For this review, use the dimensioned drawing (mm, ordinates from the lowest corner) and the shaded views. A direction names the side the tool comes from. Round coordinates to 2 decimals unless told otherwise and drop trailing zeros. Write each loop counter-clockwise with the first axis right and the second up, starting at its lowest first coordinate (ties: lowest second). Pieces come first, ordered by that corner, then holes. Notation, with made-up numbers: M 63.25,37 L 75.25,37 A27 cw 75.25,54 Z; hole C 51,-32.5 d6. An arc over 180 degrees is marked long. Write each question's results on one line, items separated by ' | '. Start each with the question number.
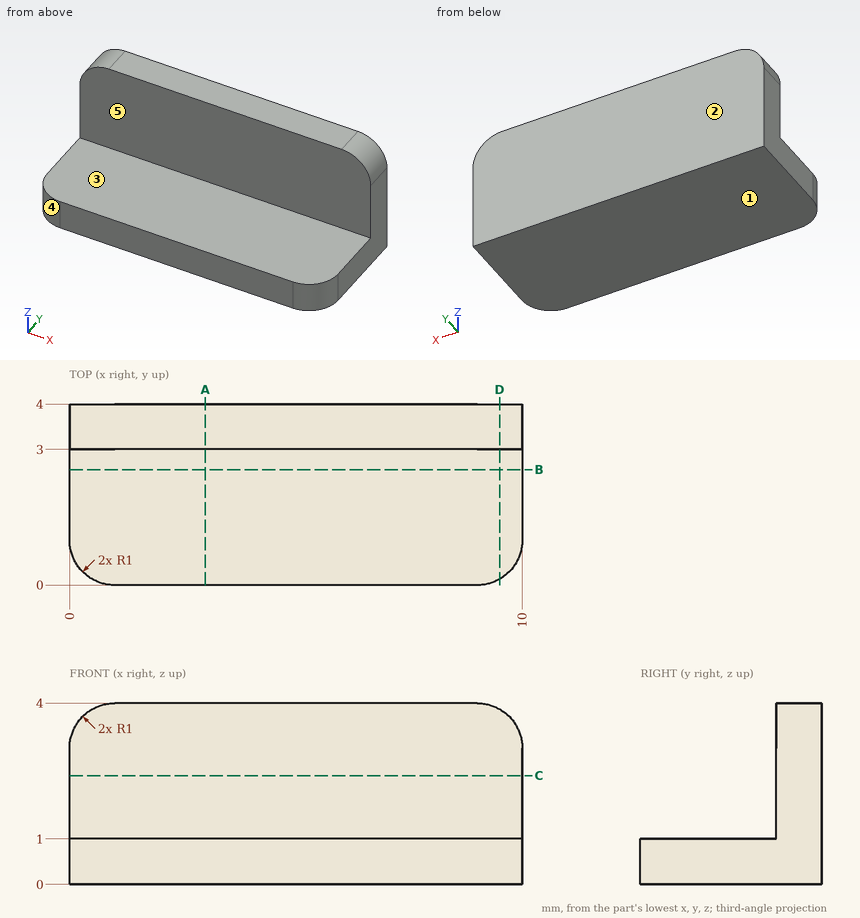
Item 1: For probe 1 along Y at (x, z) = (5, 1.15); probe 2 along Z at (x, y) = (3.75, 2.05), list the stretches that pass through material, from the lowest coordinate up.
Item 2: Mouldability with a two-part tool opening along Z and no side actions: class the marked faces 1, 2 and 3 as pulls with the +Z half, pulls with the -Z half, needs draft (parallel to the pull), parting line crosses it, or undercut.
Item 3: We need section A-A on x = 3. State the section outline as (y, z) points.
Item 4: We need section B-B on y = 2.55. State the section outline as (x, z) points, then the cut area to 3 significant figures.
Item 5: We need section C-C on z = 2.4. State the section outline as (x, y) points, then the cut area to 3 significant figures.
Item 6: For the marked faces 4 and 5, list the 3-axis set-ups (+Z, -Z, +X, -X, +Y, -Y) from which the entire face can be reached by the end or side of a thin tool; tool diameter is ignored.
Item 7: Insertion check: P1, Ø1.5, axis at x = 4, y = 2, coming from the +Z side. The pin has a flat end and moves straight along its axis. Give the tip position at first contact, or say it passes through.
Item 8: We need section D-D on x = 9.5. State the section outline as (y, z) points, then the cut area to 3 significant figures.
Numbers:
1) probe 1: y = 3 to 4 | probe 2: z = 0 to 1
2) face 1: pulls with the -Z half | face 2: needs draft | face 3: pulls with the +Z half
3) outline: M 0,0 L 4,0 L 4,4 L 3,4 L 3,1 L 0,1 Z
4) outline: M 0,0 L 10,0 L 10,1 L 0,1 Z | area: 10.0 mm^2
5) outline: M 0,3 L 10,3 L 10,4 L 0,4 Z | area: 10.0 mm^2
6) face 4: +Z, -Z, -X, -Y | face 5: +Z, +X, -X, -Y
7) P1: stops at z = 1
8) outline: M 0.13,0 L 4,0 L 4,3.87 L 3,3.87 L 3,1 L 0.13,1 Z | area: 6.73 mm^2
